The figure shows three views and two pictorial views of one solid part (mm, origin at its lowest corner). Answer the questions. A direction names the side the tool comes from. Coordinates: 2 decimals unless noted, no trailing zeros. Order: outer loops, then holes, each group sorted by start corner. A loop starts at its lowest first (then second) coordinate and runs counter-clockwise, first axis right, second up. Notation, with made-up numbers: (-23.5, -26) -> (32.5, -26) arc R14 cw to (32.5, -21) -> close; hole circle Ø7 at (-21.75, 3). An arc over 180 degrees is marked (long way). Return JSON: item names as keys, results as strings.
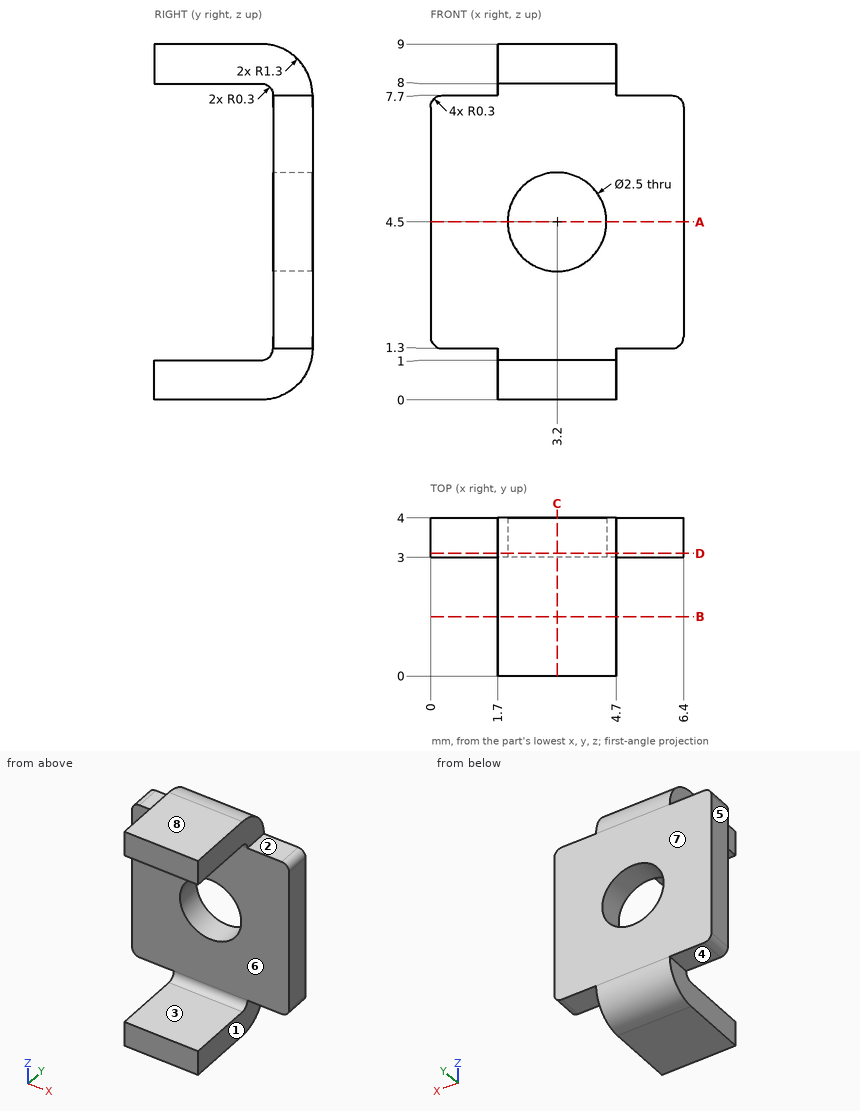
Item 1: Determine the mould class of the marked faces 6, 7 and 8 for opening direction Z: pulls with the +Z half, pulls with the -Z half, needs draft (parallel to the pull), parting line crosses it, or undercut.
Answer list:
{"face 6": "undercut", "face 7": "needs draft", "face 8": "pulls with the +Z half"}
Item 2: The part is cut by section C-C on x = 3.2. Determine the outline of the cut face in (y, z).
Answer list:
{"outline": "(0, 0) -> (2.7, 0) arc R1.3 ccw to (4, 1.3) -> (4, 3.25) -> (3, 3.25) -> (3, 1.3) arc R0.3 cw to (2.7, 1) -> (0, 1) -> close; (0, 8) -> (2.7, 8) arc R0.3 cw to (3, 7.7) -> (3, 5.75) -> (4, 5.75) -> (4, 7.7) arc R1.3 ccw to (2.7, 9) -> (0, 9) -> close"}
Item 3: Find the intervals of material crossed by probe 1 along X at (y, z) = (3.8, 4.5); probe 2 along Z at (x, y) = (2.25, 2.65); probe 3 along Z at (x, y) = (6, 3.6), in increasing order.
Answer list:
{"probe 1": "0 to 1.95, 4.45 to 6.4", "probe 2": "0 to 1, 8 to 9", "probe 3": "1.3 to 7.7"}
Item 4: The part is cut by section D-D on y = 3.1. Determine the outline of the cut face in (x, z).
Answer list:
{"outline": "(0, 1.6) arc R0.3 ccw to (0.3, 1.3) -> (1.7, 1.3) -> (1.7, 0.06) -> (4.7, 0.06) -> (4.7, 1.3) -> (6.1, 1.3) arc R0.3 ccw to (6.4, 1.6) -> (6.4, 7.4) arc R0.3 ccw to (6.1, 7.7) -> (4.7, 7.7) -> (4.7, 8.94) -> (1.7, 8.94) -> (1.7, 7.7) -> (0.3, 7.7) arc R0.3 ccw to (0, 7.4) -> close; hole circle Ø2.5 at (3.2, 4.5)"}
Item 5: The part is cut by section B-B on y = 1.5. Determine the outline of the cut face in (x, z).
Answer list:
{"outline": "(1.7, 0) -> (4.7, 0) -> (4.7, 1) -> (1.7, 1) -> close; (1.7, 8) -> (4.7, 8) -> (4.7, 9) -> (1.7, 9) -> close"}
Item 6: Which of the six approach directions +Z, -Z, +X, -X, +Y, -Y give full straight-line access (tool end or side, diameter ignored) to the marked faces 1, 2, 3, 4 and 5?
Answer list:
{"face 1": "-Z, +X, +Y, -Y", "face 2": "+Z, +X, +Y, -Y", "face 3": "+X, -X, -Y", "face 4": "-Z, -X, +Y, -Y", "face 5": "+Z, -Z, -X, +Y, -Y"}
Item 7: Flat-ended cylindrical pins translate along their axes: pin 1 (1.1 mm diameter, centred on x = 1, y = 3.5, fed in from -Z); pin 2 (1.9 mm diameter, centred on x = 4, z = 4.5, fed in from -Y); pin 3 (1 mm diameter, centred on y = 2.5, z = 1, fed in from +X); pin 4 (2 mm diameter, centred on y = 2.5, z = 4.5, fed in from -X). Find the tip coordinate at first contact, or state that the pin passes through.
Answer list:
{"pin 1": "z = 1.3", "pin 2": "y = 3", "pin 3": "x = 4.7", "pin 4": "x = 0"}
Item 8: The part is cut by section A-A on z = 4.5. Determine the outline of the cut face in (x, y).
Answer list:
{"outline": "(0, 3) -> (1.95, 3) -> (1.95, 4) -> (0, 4) -> close; (4.45, 3) -> (6.4, 3) -> (6.4, 4) -> (4.45, 4) -> close"}
